Geometry check sheet. Reference: drawing and pictorial views, mm from the part's lowest x, y, z. Round coordinates to 2 decimals unless told otherwise and drop trailing zeros. Order: outer loops, then holes, each group sorted by start corner. A loop starts at its lowest first (then second) coordinate and runs counter-clockwise, first axis right, second up.
(1) Sectioned sample at C-C (x = 521). Record the boundary of the cut face in (y, z), plus the area to 3 significant figures.
(2) Sectioned sample at B-B (y = 804.5). Record the boundary of the cut face in (x, z), plus the area to 3 significant figures.
(3) Material ranges on line 1 along Z through (x, y) = (1781, 396.5); line 2 along X through (y, z) = (350, 501.5); line 3 along X through (y, z) = (1047.5, 489.5), recorded low to high.
(4) Go/stop test with flat-tipped pins: pin 1 (5 mm diameter, centred on x = 548, y = 274.5, fed in from +Z); pin 2 (22.5 mm diameter, centred on y = 455.5, z = 536, fed in from +X); pin 3 (12 mm diameter, centred on x = 400.5, y = 786, fed in from +Z). Record where each tip stops, or that it passes through.
(5) Sectioned sample at A-A (x = 203.5). Record the boundary of the cut face in (y, z), plus the area to 3 significant figures.
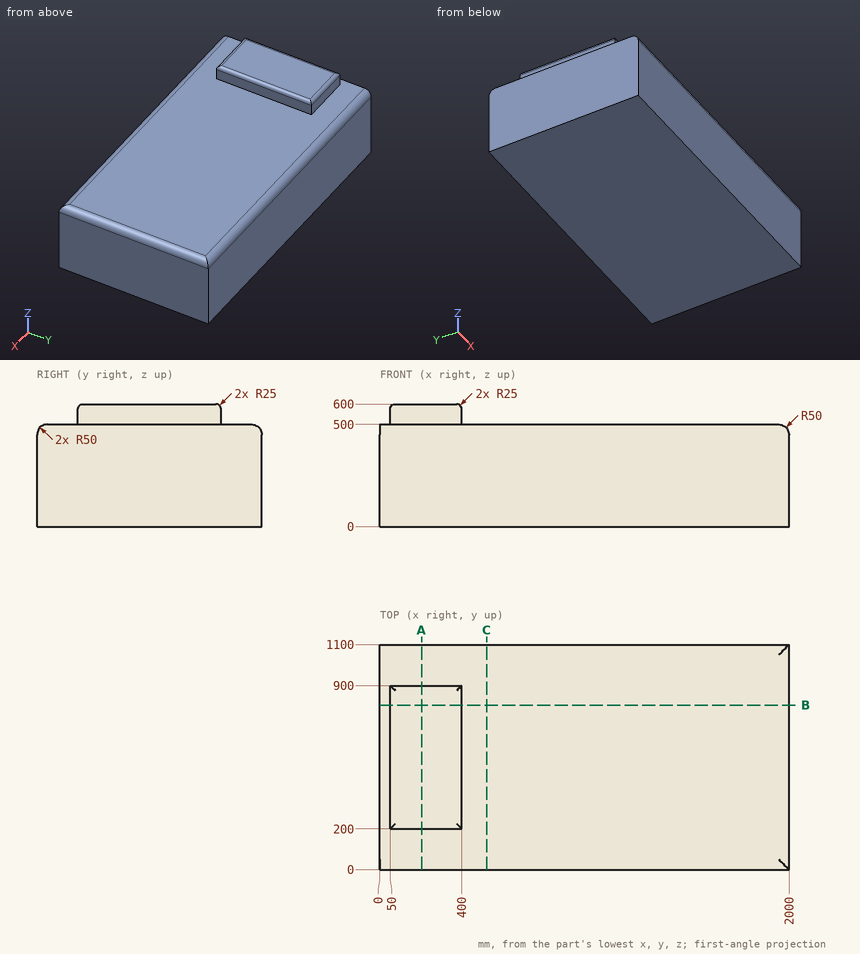
Answer below:
1. outline: (0, 0) - (1100, 0) - (1100, 450) arc R50 ccw to (1050, 500) - (50, 500) arc R50 ccw to (0, 450) - close
1. area: 549,000 mm2
2. outline: (0, 0) - (2000, 0) - (2000, 450) arc R50 ccw to (1950, 500) - (400, 500) - (400, 575) arc R25 ccw to (375, 600) - (75, 600) arc R25 ccw to (50, 575) - (50, 500) - (0, 500) - close
2. area: 1,030,000 mm2
3. line 1: z = 0 to 500
3. line 2: x = 50 to 400
3. line 3: x = 0 to 1980.66
4. pin 1: stops at z = 500
4. pin 2: stops at x = 400
4. pin 3: stops at z = 590.64
5. outline: (0, 0) - (1100, 0) - (1100, 450) arc R50 ccw to (1050, 500) - (900, 500) - (900, 575) arc R25 ccw to (875, 600) - (225, 600) arc R25 ccw to (200, 575) - (200, 500) - (50, 500) arc R50 ccw to (0, 450) - close
5. area: 619,000 mm2
